Build history of the part. All positions in model axes, mm. Give positions to 0.01 mm unless a question says otherwise; leave off trailing zeros. Write each loop counter-clockwise with the first axis right and the second up, starting at its lowest first coordinate (ties: lowest second). Pieces come first, ordered by that corner, then holes.
from build123d import *

# Parameters (mm, degrees)
F0_W          = 60
F0_H          = 10
F1_DEPTH      = 2
F2_R          = 4.99999
F3_R          = 5
F4_DEPTH      = 1
F5_W          = 5
F5_H          = 3
F6_DEPTH      = 1.001
F6_DEPTH_BACK = 2.001
F7_R          = 2
F8_DEPTH      = 2.001


# Not quite as in the source:
# - a fillet or chamfer is up to 0.001 mm smaller than in the source, because OpenCascade refuses the exact size


with BuildPart() as f1:
    # F0 (on Top) → F1 (new body)
    with BuildSketch(Plane.XY):
        with Locations((30, -5)):
            Rectangle(F0_W, F0_H)
    extrude(amount=F1_DEPTH)

    # F2 (radius 5 in the source; OpenCascade refuses exactly that, so slightly less here)
    f2_edges = [f1.edges().sort_by_distance(p)[0] for p in [
        (0, -10, 1),
        (0, 0, 1),
        (60, -10, 1),
        (60, 0, 1),
    ]]
    fillet(f2_edges, radius=F2_R)

    # F3 (on face) → F4 (join)
    with BuildSketch(Plane.XY.offset(2)):
        with Locations((5, -5)):
            Circle(F3_R)
    extrude(amount=F4_DEPTH)

    # F5 (on face) → F6 (cut, two sides)
    with BuildSketch(Plane.XY.offset(2)) as f6_sk:
        with Locations((5, -5)):
            Rectangle(F5_W, F5_H)
    extrude(amount=F6_DEPTH, mode=Mode.SUBTRACT)
    extrude(f6_sk.sketch, amount=-F6_DEPTH_BACK, mode=Mode.SUBTRACT)

    # F7 (on face) → F8 (cut, through all)
    with BuildSketch(Plane.XY.offset(2)):
        with Locations((55, -5)):
            Circle(F7_R)
    extrude(amount=-F8_DEPTH, mode=Mode.SUBTRACT)


solid = f1.part
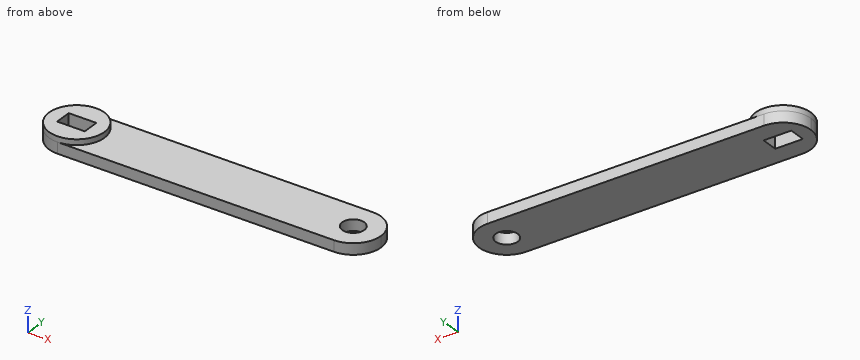
(1) Saw through at B-B, the plane y = -5.75. List the corners of the cut face in (x, z).
(2) Probe line 1 (Y direction, x = 55, z = 0.55); line 2 (Z direction, x = 53, y = -9.5); line 3 (X direction, y = -2, z = 2.8). List the from-to ranges inside material, lowest first.
(3) Saw through at D-D, the plane y = -2.5. List the corners of the cut face in (x, z), plus the area to 3 significant figures.
(4) Saw through at A-A, the plane z = 1.2. Give the number of separate pieces and of enclosed holes in the cut face, plus the area to 3 significant figures.
(5) Saw through at C-C, the plane x = 9. List the corners of the cut face in (y, z).
(6) Drop flat-ended pins along their axis: pin 1 (1.5 mm diameter, centred on y = -2.5, z = 2, fed in from -X); pin 2 (3 mm diameter, centred on x = 35.5, y = -6.5, fed in from +Z); pin 3 (1 mm diameter, centred on y = -2, z = 2, fed in from +X); pin 4 (2.5 mm diameter, centred on x = 55, y = -5, fed in from +Z). Give the stop position or say it passes through.
Computed values:
1. outline: (0.06, 0) - (2.5, 0) - (2.5, 3) - (0.06, 3) - close; (7.5, 0) - (53.15, 0) - (53.15, 2) - (9.94, 2) - (9.94, 3) - (7.5, 3) - close; (56.85, 0) - (59.94, 0) - (59.94, 2) - (56.85, 2) - close
2. line 1: y = -10 to -7, -3 to 0
2. line 2: z = 0 to 2
2. line 3: x = 1 to 9
3. outline: (0.67, 0) - (59.33, 0) - (59.33, 2) - (9.33, 2) - (9.33, 3) - (0.67, 3) - close
3. area: 126 mm2
4. separate pieces: 1
4. enclosed holes: 2
4. area: 551 mm2
5. outline: (-10, 0) - (0, 0) - (0, 2) - (-2, 2) - (-2, 3) - (-8, 3) - (-8, 2) - (-10, 2) - close
6. pin 1: stops at x = 0.32
6. pin 2: stops at z = 2
6. pin 3: stops at x = 59.33
6. pin 4: passes through
